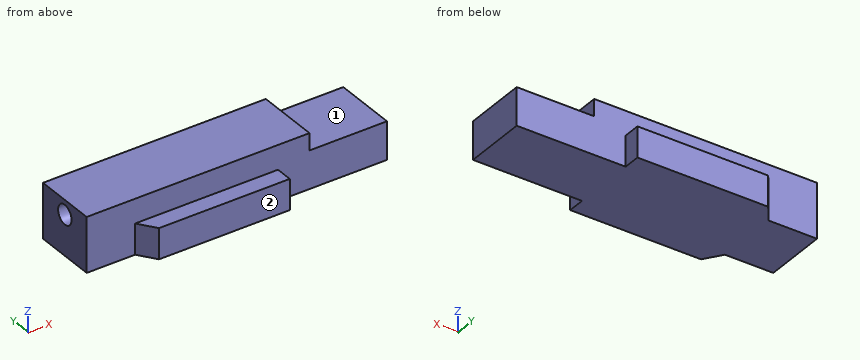
```python
from build123d import *

# Parameters (mm, degrees)
F1_DEPTH      = 12.7
F1_DEPTH_BACK = 12.7
F3_D          = 5.08
F3_DEPTH      = 5.08
F3_TIP        = 1.5261859723
F5_DEPTH      = 92
F4_W          = 8.255
F4_H          = 4.445
F6_DEPTH      = 14.352
F8_W          = 20.32
F8_H          = 4.445
F9_DEPTH      = 9.907
F10_W         = 4.445
F10_H         = 6.35
F11_DEPTH     = 50.166


# Not quite as in the source:
# - an extrude ends at something that could not be found from the text; its depth is read off the source's solid
# - a pattern or mirror of a feature is missing from the dataset's text; its kind, count and spacing are read off the source's solid


with BuildPart() as f1:
    # F0 (on Front) → F1 (new body, two sides)
    with BuildSketch(Plane.XZ) as f1_sk:
        Polygon((-39.37, 14.351), (-39.37, 0), (39.37, 0), (39.37, 9.906), (19.05, 9.906), (19.05, 14.351), align=None)
    extrude(amount=F1_DEPTH)
    extrude(f1_sk.sketch, amount=-F1_DEPTH_BACK)

    # F3
    with Locations(Plane(origin=(-39.37, 0, 0), x_dir=(0, -1, 0), z_dir=(-1, 0, 0))):
        with Locations((0, 10.541)):
            Hole(F3_D / 2, depth=F3_DEPTH)
            with Locations((0, 0, -(F3_DEPTH + F3_TIP / 2))):  # 118° drill point
                Cone(0, F3_D / 2, F3_TIP, mode=Mode.SUBTRACT)

    # F5 (cut, through all): a face of the model
    f5_faces = [f1.faces().sort_by_distance(p)[0] for p in [
        (0, 0, 0),
    ]]
    extrude(f5_faces, amount=F5_DEPTH, mode=Mode.SUBTRACT)

    # F4 (on face) → F6 (cut, through all)
    with BuildSketch(Plane.XY.offset(14.351)):
        Polygon((-39.37, 12.7), (-39.37, 8.255), (-26.67, 8.255), (-23.495, 12.7), align=None)
        with Locations((14.9225, 10.4775)):
            Rectangle(F4_W, F4_H)
    extrude(amount=-F6_DEPTH, mode=Mode.SUBTRACT)

    # F7: F1 across plane


with BuildPart() as f1_1:
    add(f1.part)
    add(f1.part.mirror(Plane.XZ), mode=Mode.INTERSECT)

    # F8 (on face) → F9 (cut, through all)
    with BuildSketch(Plane.XY.offset(9.906)):
        with Locations((29.21, -10.4775)):
            Rectangle(F8_W, F8_H)
        with Locations((29.21, 10.4775)):
            Rectangle(F8_W, F8_H)
    extrude(amount=-F9_DEPTH, mode=Mode.SUBTRACT)

    # F10 (on face) → F11 (cut, through all)
    with BuildSketch(Plane.YZ.offset(10.795)):
        with Locations((10.4775, 11.176)):
            Rectangle(F10_W, F10_H)
    f11 = extrude(amount=-F11_DEPTH, mode=Mode.SUBTRACT)

    # F11_copies: F11 across plane
    add(f11.mirror(Plane(origin=(0, 0, 0), x_dir=(0, 0, -1), z_dir=(0, -1, 0))), mode=Mode.SUBTRACT)


solid = f1_1.part
```
The listing builds one solid part. Answer for the finished solid, in the listing's coordinates (mm). Face numbers are marked on the shaded views. A direction names the side the tool comes from. Coordinates: 2 decimals unless noted, no trailing zeros. Write each loop counter-clockwise with the first axis right and the second up, starting at its lowest first coordinate (ties: lowest second). Pieces come first, ordered by that corner, then holes. Notation, with made-up numbers: (-8, 56.25) - (-1, 56.25) arc R29 cw to (-1, 89.25) - close; hole circle Ø1 at (-13.75, -22). An arc over 180 degrees is marked (long way). Return JSON: item names as keys, results as strings. Group by question number.
Q1. Which of the six approach directions +Z, -Z, +X, -X, +Y, -Y give full straight-line access (tool end or side, diameter ignored) to the marked faces 1 and 2?
Q2. The part is cut by section C-C on y = -7.5. Write down the section's boundary in (x, z).
Q3. Find the intervals of material crossed by line 1 along X through (y, z) = (-3.25, 12.75); line 2 along Z through (x, y) = (-38.3, 0); line 3 along Y through (x, z) = (-20.5, 10) (3 decimals), in increasing order. Write a range as [from, to].
Q4. Flat-ended cylindrical pins translate along their axes: pin 1 Ø13 at (x, y) = (32, -2.5) entering from +Z; pin 2 Ø8 at (x, z) = (24.5, 3.5) entering from +Y (3 decimals); pin 3 Ø7 at (x, z) = (-2, 9.5) entering from +Y; pin 4 Ø3 at (y, z) = (0, 10.541) entering from -X. Find the tip coordinate at first contact, or state that the pin passes through.
Q5. The part is cut by section A-A on z = 6. Write down the section's boundary in (x, y) (3 decimals), and give its area (3 significant figures).
Q6. The part is cut by section B-B on x = -20. Write down the section's boundary in (y, z) (3 decimals).
Q7. The part is cut by section D-D on x = 23. Write down the section's boundary in (y, z) (3 decimals), and give its area (3 significant figures).
Evaluation:
{
 "1": {"face 1": "+Z, +X, +Y, -Y", "face 2": "+Z, -Z, +X, -X, -Y"},
 "2": {"outline": "(-39.37, 0) - (39.37, 0) - (39.37, 9.91) - (19.05, 9.91) - (19.05, 14.35) - (-39.37, 14.35) - close"},
 "3": {"line 1": "x = [-39.37, 19.05]", "line 2": "z = [0, 8], [13.08, 14.35]", "line 3": "y = [-8.255, 8.255]"},
 "4": {"pin 1": "stops at z = 9.91", "pin 2": "stops at y = 8.255", "pin 3": "stops at y = 12.7", "pin 4": "stops at x = -33.67"},
 "5": {"outline": "(-39.37, -8.255) - (-26.67, -8.255) - (-23.495, -12.7) - (10.795, -12.7) - (10.795, -8.255) - (39.37, -8.255) - (39.37, 8.255) - (10.795, 8.255) - (10.795, 12.7) - (-23.495, 12.7) - (-26.67, 8.255) - (-39.37, 8.255) - close", "area": "1,620 mm2"},
 "6": {"outline": "(-12.7, 0) - (12.7, 0) - (12.7, 8.001) - (8.255, 8.001) - (8.255, 14.351) - (-8.255, 14.351) - (-8.255, 8.001) - (-12.7, 8.001) - close"},
 "7": {"outline": "(-8.255, 0) - (8.255, 0) - (8.255, 9.906) - (-8.255, 9.906) - close", "area": "164 mm2"}
}
